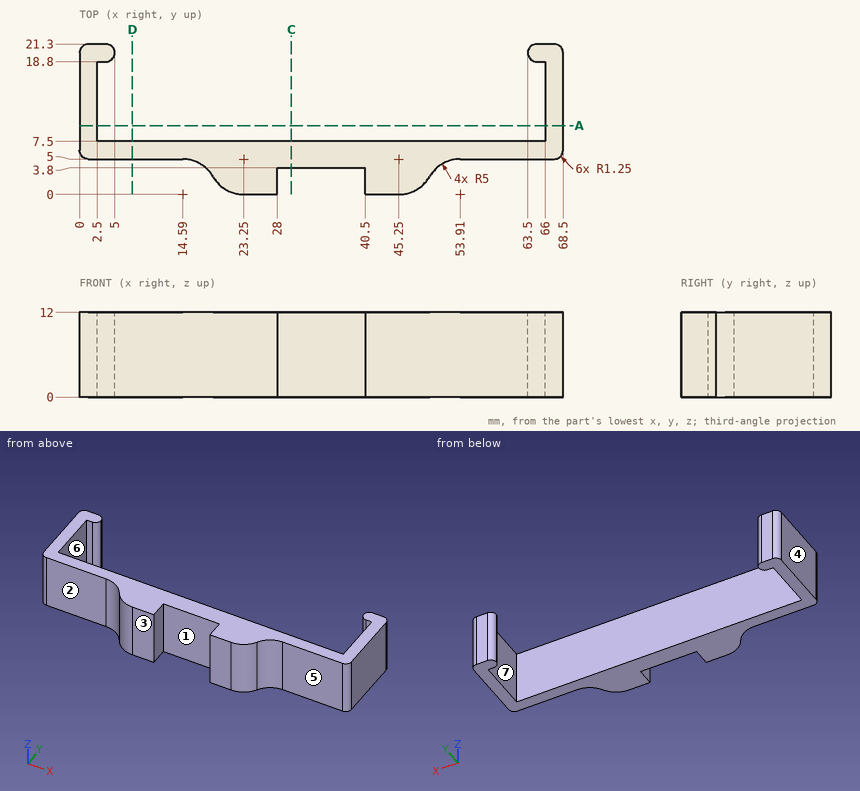
Job drawing, mm, ordinate dimensions from the low corner. One solid piece. A direction names the side the tool comes from. Coordinates: 2 decimals unless noted, no trailing zeros. Order: outer loops, then holes, each group sorted by start corner. A loop starts at its lowest first (then second) coordinate and runs counter-clockwise, first axis right, second up. Notation, with made-up numbers: (58.5, 79) -> (94.5, 79) arc R23 ccw to (94.5, 98) -> close; hole circle Ø9 at (53, 35.5). An arc over 180 degrees is marked (long way). Return JSON: item names as keys, results as strings. Group by question number.
Item 1: Tool access for the marked faces 1, 2 and 3: list every direction of +Z, -Z, +X, -X, +Y, -Y with a clear straight run to the whole face (end or side of a thin tool).
Item 2: Saw through at C-C on x = 30. Write the cut outline in (y, z).
Item 3: Wall check: line 1 along X through (y, z) = (11.5, 6.5); line 2 along Y through (x, z) = (13, 9.5); line 3 along X through (y, z) = (3.5, 6.5). Give the ranges that are in metal, low to high. Write a range as [from, to].
Item 4: Saw through at D-D on x = 7.5. Write the cut outline in (y, z).
Item 5: Saw through at A-A on y = 9.75. Write the cut outline in (x, z).
Item 6: Flat gauge pins, fed straight in: P1, Ø0.6, axis at x = 3.5, z = 6, coming from the -Y side; P2, Ø10, axis at x = 35, y = 13.5, coming from the -Z side; P3, Ø6, axis at x = 33, z = 3.5, coming from the -Y side; P4, Ø4, axis at x = 30.5, z = 5.5, coming from the +Y side. Where does each tip first touch, or does it go through?
Item 7: Pull direction Y, two halves, no side cores. Call the marked faces 4, 5, 6 and 7: pulls with the +Y half, pulls with the -Y half, needs draft (parallel to the pull), parting line crosses it, or undercut.
Values found:
{
 "1": {"face 1": "+Z, -Z, -Y", "face 2": "+Z, -Z, -X, -Y", "face 3": "+Z, -Z, +X, -X, -Y"},
 "2": {"outline": "(3.8, 0) -> (7.5, 0) -> (7.5, 12) -> (3.8, 12) -> close"},
 "3": {"line 1": "x = [0, 2.5], [66, 68.5]", "line 2": "y = [5, 7.5]", "line 3": "x = [18.16, 28], [40.5, 50.34]"},
 "4": {"outline": "(5, 0) -> (7.5, 0) -> (7.5, 12) -> (5, 12) -> close"},
 "5": {"outline": "(0, 0) -> (2.5, 0) -> (2.5, 12) -> (0, 12) -> close; (66, 0) -> (68.5, 0) -> (68.5, 12) -> (66, 12) -> close"},
 "6": {"P1": "stops at y = 5", "P2": "passes through", "P3": "stops at y = 3.8", "P4": "stops at y = 7.5"},
 "7": {"face 4": "needs draft", "face 5": "pulls with the -Y half", "face 6": "undercut", "face 7": "undercut"}
}
